Check sheet for the modelled part. Datum: model origin and axes. Units: mm. Face numbers are marked on the shaded views. A direction names the side the tool comes from. Round coordinates to 2 decimals unless told otherwise and drop trailing zeros. Order: outer loops, then holes, each group sorted by start corner. A loop starts at its lowest first (then second) coordinate and runs counter-clockwise, first axis right, second up.
Q1. Mould release check, pull along Y, two halves, no side actions. Record for the marked faces 1, 2, 3 and 4: +Y half, -Y half, draft (parallel to the pull), parting line (faces both ways), or undercut.
Q2. Depth check by flat-ended pin: P1, Ø8, axis at y = -35.03, z = 12.8, coming from the -X side; P2, Ø1.5, axis at x = -17, z = 18.5, coming from the +Y side; P3, Ø4.5, axis at x = 28.5, z = 7.5, coming from the +Y side. Enter the tip coordinate at first touch or a pass-through.
Q3. Cross-section at B-B on y = -73.5. Record the cut outline in (x, z).
Q4. Cross-section at A-A on y = -51. Record the cut outline in (x, z).
Q5. Scan lines: probe 1 along X at (y, z) = (-59, 15.5); probe 2 along X at (y, z) = (-41.5, 13.75); probe 3 along X at (y, z) = (-13.5, 7). Record each from-to range of solid material in increasing order.
Q6. Set-up check for the marked faces 5, 6 and 7: record each of +Z, -Z, +X, -X, +Y, -Y from which the full face is reachable in a straight line by a thin tool's end or side.
Q7. Cross-section at C-C on y = -22. Record the cut outline in (x, z).
from build123d import *

# Parameters (mm, degrees)
F1_DEPTH = 25.4
F2_R     = 6.722416
F3_DEPTH = 19.304


with BuildPart() as f1:
    # F0 (on Top) → F1 (new body)
    with BuildSketch(Plane.XY):
        Polygon((-22.084782, 21.292763), (-18.868631, 22.704166), (-22.891159, 29.745255), (-35.822235, 29.745255), (-22.417855, 74.350529), (-43.49843, 29.745255), (-35.822235, 22.704166), (-25.267471, 22.704166), align=None)
        Polygon((-22.084782, 13.950433), (-22.084782, 18.870648), (-43.49843, 18.870648), (-48.935734, 26.866684), (-40.300015, 51.81431), (-56.316686, 29.745255), (-52.134149, 18.870648), (-43.49843, 13.950433), align=None)
        Polygon((-22.084782, 6.608103), (-22.084782, 11.514296), (-37.421443, 11.514296), (-55.012722, -4.994443), (-59.383125, -0.337456), (-64.927801, -13.113492), (-28.785726, -94.673045), (-55.012722, -13.113492), (-37.421443, 6.608103), align=None)
        Polygon((-16.357765, 3.304051), (-22.084782, 6.608103), (-32.656161, -5.243477), (-38.534627, 0), (-42.777374, -7.354087), (-16.357765, -100.430191), (-32.656161, -14.804116), align=None)
        Polygon((-14.944169, 24.426411), (-11.042391, 26.138701), (-14.944169, 32.623827), align=None)
        Polygon((7.062444, 31.984143), (7.062444, 27.885296), (11.042391, 26.138701), align=None)
        Polygon((7.062444, 27.885296), (0, 30.98464), (-7.062444, 27.885296), (-11.042391, 26.138701), (-14.944169, 24.426411), (-18.868631, 22.704166), (-22.084782, 21.292763), (-22.084782, 18.870648), (-22.084782, 13.950433), (-22.084782, 11.514296), (-22.084782, 6.608103), (-16.357765, 3.304051), (-10.630748, 0), (-17.385691, -17.181048), (-5.11746, -53.733349), (0, -56.685733), (5.11746, -53.733349), (17.385691, -17.181048), (10.630748, 0), (16.357765, 3.304051), (22.084782, 6.608103), (22.084782, 11.514296), (22.084782, 13.950433), (22.084782, 18.870648), (22.084782, 21.292763), (18.868631, 22.704166), (15.330053, 24.257066), (11.042391, 26.138701), align=None)
        Polygon((-11.042391, 26.138701), (-7.062444, 27.885296), (-7.062444, 32.623827), align=None)
        Polygon((13.88838, 32.623827), (11.042391, 26.138701), (15.330053, 24.257066), align=None)
        Polygon((22.891159, 29.745255), (18.868631, 22.704166), (22.084782, 21.292763), (25.267471, 22.704166), (35.822235, 22.704166), (43.49843, 29.745255), (22.417855, 74.350529), (35.822235, 29.745255), align=None)
        Polygon((43.49843, 18.870648), (22.084782, 18.870648), (22.084782, 13.950433), (43.49843, 13.950433), (52.134149, 18.870648), (56.316686, 29.745255), (40.300015, 51.81431), (48.935734, 26.866684), align=None)
        Polygon((37.421443, 11.514296), (22.084782, 11.514296), (22.084782, 6.608103), (37.421443, 6.608103), (55.012722, -13.113492), (28.785726, -94.673045), (64.927801, -13.113492), (59.383125, -0.337456), (55.012722, -4.994443), align=None)
        Polygon((32.656161, -5.243477), (22.084782, 6.608103), (16.357765, 3.304051), (32.656161, -14.804116), (16.357765, -100.430191), (42.777374, -7.354087), (38.534627, 0), align=None)
    extrude(amount=F1_DEPTH)

    # F2 (on Right) → F3 (cut, symmetric)
    with BuildSketch(Plane.YZ):
        with Locations((-35.03409, 12.8016)):
            Circle(F2_R)
    extrude(amount=F3_DEPTH, both=True, mode=Mode.SUBTRACT)


solid = f1.part
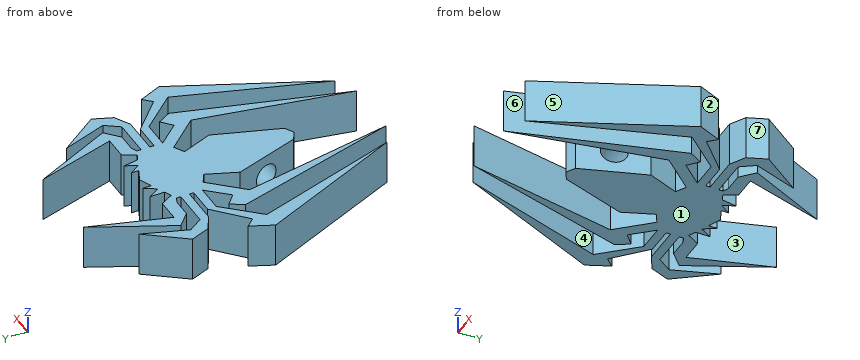
Results found:
1. face 1: draft
1. face 2: +Y half
1. face 3: undercut
1. face 4: undercut
2. P1: stops at x = -56.99
2. P2: stops at y = 23.85
2. P3: stops at y = 66.24
3. outline: (-38.17, 0) - (-35.59, 0) - (-35.59, 25.4) - (-38.17, 25.4) - close; (-24, 0) - (-21.48, 0) - (-21.48, 25.4) - (-24, 25.4) - close; (21.48, 0) - (24, 0) - (24, 25.4) - (21.48, 25.4) - close; (35.59, 0) - (38.17, 0) - (38.17, 25.4) - (35.59, 25.4) - close
4. outline: (-48.14, 0) - (-42.83, 0) - (-42.83, 25.4) - (-48.14, 25.4) - close; (-30.39, 0) - (-25.77, 0) - (-25.77, 25.4) - (-30.39, 25.4) - close; (-6.03, 0) - (6.03, 0) - (6.03, 25.4) - (-6.03, 25.4) - close; (25.77, 0) - (30.39, 0) - (30.39, 25.4) - (25.77, 25.4) - close; (42.83, 0) - (48.14, 0) - (48.14, 25.4) - (42.83, 25.4) - close
5. probe 1: x = -44.59 to -40.26, -28.12 to -24.24, 24.24 to 28.12, 40.26 to 44.59
5. probe 2: x = -52.35 to -45.88, -33.09 to -27.57, 27.57 to 33.09, 45.88 to 52.35
5. probe 3: x = -64.76 to -54.89, -41.03 to -31.48, -15.94 to 15.94, 31.48 to 41.03, 54.89 to 64.76
6. face 5: +Z, -Z, +X, -Y
6. face 6: +Z, -Z
6. face 7: +Z, -Z, +X
7. outline: (-60.99, 0) - (-52.16, 0) - (-52.16, 25.4) - (-60.99, 25.4) - close; (-38.62, 0) - (-31.29, 0) - (-31.29, 25.4) - (-38.62, 25.4) - close; (-15.77, 0) - (15.77, 0) - (15.77, 25.4) - (-15.77, 25.4) - close; (31.29, 0) - (38.62, 0) - (38.62, 25.4) - (31.29, 25.4) - close; (52.16, 0) - (60.99, 0) - (60.99, 25.4) - (52.16, 25.4) - close
